Part model, mm, in its own coordinate system. A direction names the side the tool comes from. Round coordinates to 2 decimals unless told otherwise and drop trailing zeros. Write each loop counter-clockwise with the first axis right and the second up, starting at its lowest first coordinate (ties: lowest second). Pieces come first, ordered by that corner, then holes.
```python
from build123d import *

# Parameters (mm, degrees)
BOSS_EXTRUDE1_DEPTH      = 38.1
BOSS_EXTRUDE1_DEPTH_BACK = 38.1
CUT_EXTRUDE1_DEPTH       = 55.4
CUT_EXTRUDE1_DEPTH_BACK  = 30
SKETCH2_R                = 4
SKETCH3_R                = 6.5
CUT_EXTRUDE2_DEPTH       = 18.2
CUT_EXTRUDE3_START       = 19
SKETCH4_W                = 24
SKETCH4_H                = 20
CUT_EXTRUDE3_DEPTH       = 10


with BuildPart() as part:
    # Sketch1 → Boss-Extrude1 (new, two sides: drawn at the far end of the back side and taken through both)
    with BuildSketch(Plane.XY.offset(-BOSS_EXTRUDE1_DEPTH_BACK)):
        with BuildLine():
            Line((-10, -15.714961024), (-10, 14.285038976))
            Line((-10, 14.285038976), (0, 14.285038976))
            Line((0, 14.285038976), (0, 1))
            ThreePointArc((0, 1), (-0.707106781, -0.707106781), (1, 0))
            Line((1, 0), (18, 0))
            Line((18, 0), (18, -3.779961024))
            Line((18, -3.779961024), (23.5, -3.779961024))
            Line((23.5, -3.779961024), (23.5, -11.899961024))
            Line((23.5, -11.899961024), (19, -11.899961024))
            Line((19, -11.899961024), (19, -15.714961024))
            Line((19, -15.714961024), (-10, -15.714961024))
        make_face()
    extrude(amount=BOSS_EXTRUDE1_DEPTH + BOSS_EXTRUDE1_DEPTH_BACK)

    # Sketch2 → Cut-Extrude1 (cut, two sides: drawn at the far end of the back side and taken through both)
    with BuildSketch(Plane(origin=(0, 0, 0), x_dir=(0, 0, -1), z_dir=(1, 0, 0)).offset(-CUT_EXTRUDE1_DEPTH_BACK)):
        with Locations((-19.05, -7.839961024)):
            Circle(SKETCH2_R)
        with Locations((19.05, -7.839961024)):
            Circle(SKETCH2_R)
    extrude(amount=CUT_EXTRUDE1_DEPTH + CUT_EXTRUDE1_DEPTH_BACK, mode=Mode.SUBTRACT)

    # Sketch3 → Cut-Extrude2 (cut)
    with BuildSketch(Plane(origin=(0, 0, 0), x_dir=(0, 0, -1), z_dir=(1, 0, 0))):
        with Locations((-19.05, -7.839961024)):
            Circle(SKETCH3_R)
        with Locations((19.05, -7.839961024)):
            Circle(SKETCH3_R)
    extrude(amount=-CUT_EXTRUDE2_DEPTH, mode=Mode.SUBTRACT)

    # Sketch4 → Cut-Extrude3 (cut)
    with BuildSketch(Plane(origin=(0, 0, 0), x_dir=(0, 0, -1), z_dir=(1, 0, 0)).offset(CUT_EXTRUDE3_START)):
        with Locations((-19.05, -7.839961024)):
            Rectangle(SKETCH4_W, SKETCH4_H)
        with Locations((19.05, -7.839961024)):
            Rectangle(SKETCH4_W, SKETCH4_H)
    extrude(amount=CUT_EXTRUDE3_DEPTH, mode=Mode.SUBTRACT)


solid = part.part
```
Q1. Mould opens along X. For faces 1 (the cylindrical face through (9.37, -5.14, -16.1)), 2 (the flat face through (23.5, -8, 0)), 3 (the cylindrical face through (-0.73, -0.683, -0.533)) say: +X half, -X half, draft (parallel to the pull), parting line (faces both ways), or undercut.
Values follow:
face 1: draft
face 2: +X half
face 3: undercut
Q2. Cut at C-C on y = -7. Write the cut outline in (x, z), plus the area to 3 significant figures.
Values follow:
outline: (-10, -38.1) - (23.5, -38.1) - (23.5, -31.05) - (19, -31.05) - (19, -22.96) - (0, -22.96) - (0, -25.5) - (-10, -25.5) - close; (-10, -12.6) - (0, -12.6) - (0, -15.14) - (19, -15.14) - (19, -7.05) - (23.5, -7.05) - (23.5, 7.05) - (19, 7.05) - (19, 15.14) - (0, 15.14) - (0, 12.6) - (-10, 12.6) - close; (-10, 25.5) - (0, 25.5) - (0, 22.96) - (19, 22.96) - (19, 31.05) - (23.5, 31.05) - (23.5, 38.1) - (-10, 38.1) - close
area: 1,780 mm2
Q3. Cut at D-D on z = -21. Write the cut outline in (x, y).
Values follow:
outline: (-10, -15.71) - (19, -15.71) - (19, -11.33) - (0, -11.33) - (0, -14.04) - (-10, -14.04) - close; (-10, -1.64) - (0, -1.64) - (0, -4.35) - (19, -4.35) - (19, -3.78) - (18, -3.78) - (18, 0) - (1, 0) arc R1 cw (long way) to (0, 1) - (0, 14.29) - (-10, 14.29) - close
Q4. Which spindle directions (+Z, -Z, +X, -X, +Y, -Y) get a long thin tool onto all of the face, cutting with end or side? Do faces 4 (the flat face through (0, -11, -16)), 5 (the flat face through (20, -3.78, -1)), 6 (the flat face through (21, -8, 7.05)). Say none if no direction does.
Values follow:
face 4: -X
face 5: +Z, -Z, +X, +Y
face 6: +X, +Y, -Y
Q5. Cut at A-A on z = 19.05. Write the cut outline in (x, y), plus the area to 3 significant figures.
Values follow:
outline: (-10, -15.71) - (19, -15.71) - (19, -11.84) - (0, -11.84) - (0, -14.34) - (-10, -14.34) - close; (-10, -1.34) - (0, -1.34) - (0, -3.84) - (19, -3.84) - (19, -3.78) - (18, -3.78) - (18, 0) - (1, 0) arc R1 cw (long way) to (0, 1) - (0, 14.29) - (-10, 14.29) - close
area: 310 mm2
Q6. Wall check: L1, parallel to Y at x = -4, z = -19; L2, parallel to Z at x = 3, y = -9.75; L3, parallel to Y at x = 10, z = 19. Give the ranges that are in metal, low to high.
Values follow:
L1: y = -15.71 to -14.34, -1.34 to 14.29
L2: z = -38.1 to -22.56, -15.54 to 15.54, 22.56 to 38.1
L3: y = -15.71 to -11.84, -3.84 to 0
Q7. Drop flat-ended pins along their axis: pin 1 (1.2 mm diameter, centred on x = 0, y = 0, fed in from -Z); pin 2 (2 mm diameter, centred on x = 20.5, z = -36, fed in from -Y); pin 3 (12 mm diameter, centred on y = -2.5, z = -15.5, fed in from +X); pin 4 (5 mm diameter, centred on x = 14, z = -23, fed in from +Y). Give the stop position or say it passes through.
Values follow:
pin 1: passes through
pin 2: stops at y = -11.9
pin 3: stops at x = 19
pin 4: stops at y = 0
Q8. Cut at B-B on z = -0.5. Write the cut outline in (x, y), plus the area to 3 significant figures.
Values follow:
outline: (-10, -15.71) - (19, -15.71) - (19, -11.9) - (23.5, -11.9) - (23.5, -3.78) - (18, -3.78) - (18, 0) - (1, 0) arc R1 cw (long way) to (0, 1) - (0, 14.29) - (-10, 14.29) - close
area: 629 mm2
